Geometry: final body of the model. Coordinates: model frame, mm. Face numbers are marked on the shaded views. A direction names the side the tool comes from. Round coordinates to 2 decimals unless told otherwise and drop trailing zeros. Order: outer loops, then holes, each group sorted by start corner. A loop starts at its lowest first (then second) coordinate and runs counter-clockwise, first axis right, second up. Notation, with made-up numbers: (-15.75, -16.75) -> (16.25, -16.75) arc R5 ccw to (16.25, -8.75) -> close; hole circle Ø4 at (-17, 27.5). An arc over 180 degrees is marked (long way). Put each result on its own line as item: value.
```python
from build123d import *

# Parameters (mm, degrees)
EXTRUDE_1_DEPTH     = 4
EXTRUDE_START       = 2
EXTRUDE_2_DEPTH     = 2
EXTRUDE_3_DEPTH     = 2
SKETCH_4_R          = 1.6
CUT_EXTRUDE_1_DEPTH = 10
CUT_EXTRUDE_2_DEPTH = 3
SKETCH_7_R          = 1.6
CUT_EXTRUDE_3_DEPTH = 10
CUT_EXTRUDE_4_DEPTH = 3


with BuildPart() as part:
    # 草图1 → 凸台-拉伸1 (new body)
    with BuildSketch(Plane.XY):
        with BuildLine():
            Line((-35.40625, 64.537081934), (4.59375, 64.537081934))
            ThreePointArc((4.59375, 64.537081934), (10.957711031, 61.901042965), (13.59375, 55.537081934))
            Line((13.59375, 55.537081934), (13.59375, 15.537081934))
            ThreePointArc((13.59375, 15.537081934), (10.957711031, 9.173120903), (4.59375, 6.537081934))
            Line((4.59375, 6.537081934), (-35.40625, 6.537081934))
            ThreePointArc((-35.40625, 6.537081934), (-41.770211031, 9.173120903), (-44.40625, 15.537081934))
            Line((-44.40625, 15.537081934), (-44.40625, 55.537081934))
            ThreePointArc((-44.40625, 55.537081934), (-41.770211031, 61.901042965), (-35.40625, 64.537081934))
        make_face()
    extrude(amount=-EXTRUDE_1_DEPTH)

    # 草图2 → 凸台-拉伸2 (add)
    with BuildSketch(Plane.XY.offset(EXTRUDE_START)):
        with BuildLine():
            Line((13.59375, 15.537081934), (13.59375, 55.537081934))
            ThreePointArc((13.59375, 55.537081934), (10.957711031, 61.901042965), (4.59375, 64.537081934))
            Line((4.59375, 64.537081934), (-35.40625, 64.537081934))
            ThreePointArc((-35.40625, 64.537081934), (-41.770211031, 61.901042965), (-44.40625, 55.537081934))
            Line((-44.40625, 55.537081934), (-44.40625, 15.537081934))
            ThreePointArc((-44.40625, 15.537081934), (-41.770211031, 9.173120903), (-35.40625, 6.537081934))
            Line((-35.40625, 6.537081934), (4.59375, 6.537081934))
            ThreePointArc((4.59375, 6.537081934), (10.957711031, 9.173120903), (13.59375, 15.537081934))
        make_face()
        with BuildLine():
            Line((-35.40625, 63.537081934), (-25.40625, 63.537081934))
            Line((-25.40625, 63.537081934), (-25.40625, 45.537081934))
            Line((-25.40625, 45.537081934), (-43.40625, 45.537081934))
            Line((-43.40625, 45.537081934), (-43.40625, 55.537081934))
            ThreePointArc((-43.40625, 55.537081934), (-41.063104249, 61.193936184), (-35.40625, 63.537081934))
        make_face(mode=Mode.SUBTRACT)
        with BuildLine():
            Line((12.59375, 55.537081934), (12.59375, 45.537081934))
            Line((12.59375, 45.537081934), (-5.40625, 45.537081934))
            Line((-5.40625, 45.537081934), (-5.40625, 63.537081934))
            Line((-5.40625, 63.537081934), (4.59375, 63.537081934))
            ThreePointArc((4.59375, 63.537081934), (10.250604249, 61.193936184), (12.59375, 55.537081934))
        make_face(mode=Mode.SUBTRACT)
        with BuildLine():
            Line((-35.40625, 7.537081934), (-25.40625, 7.537081934))
            Line((-25.40625, 7.537081934), (-25.40625, 25.537081934))
            Line((-25.40625, 25.537081934), (-43.40625, 25.537081934))
            Line((-43.40625, 25.537081934), (-43.40625, 15.537081934))
            ThreePointArc((-43.40625, 15.537081934), (-41.063104249, 9.880227685), (-35.40625, 7.537081934))
        make_face(mode=Mode.SUBTRACT)
        with BuildLine():
            Line((-5.40625, 25.537081934), (12.59375, 25.537081934))
            Line((12.59375, 25.537081934), (12.59375, 15.537081934))
            ThreePointArc((12.59375, 15.537081934), (10.250604249, 9.880227685), (4.59375, 7.537081934))
            Line((4.59375, 7.537081934), (-5.40625, 7.537081934))
            Line((-5.40625, 7.537081934), (-5.40625, 25.537081934))
        make_face(mode=Mode.SUBTRACT)
    extrude(amount=-EXTRUDE_2_DEPTH)

    # 草图3 → 凸台-拉伸3 (add)
    with BuildSketch(Plane.XY.offset(2).offset(EXTRUDE_START)):
        with BuildLine():
            Line((13.59375, 15.537081934), (13.59375, 55.537081934))
            ThreePointArc((13.59375, 55.537081934), (10.957711031, 61.901042965), (4.59375, 64.537081934))
            Line((4.59375, 64.537081934), (-35.40625, 64.537081934))
            ThreePointArc((-35.40625, 64.537081934), (-41.770211031, 61.901042965), (-44.40625, 55.537081934))
            Line((-44.40625, 55.537081934), (-44.40625, 15.537081934))
            ThreePointArc((-44.40625, 15.537081934), (-41.770211031, 9.173120903), (-35.40625, 6.537081934))
            Line((-35.40625, 6.537081934), (4.59375, 6.537081934))
            ThreePointArc((4.59375, 6.537081934), (10.957711031, 9.173120903), (13.59375, 15.537081934))
        make_face()
        with BuildLine():
            Line((-43.40625, 55.537081934), (-43.40625, 45.537081934))
            Line((-43.40625, 45.537081934), (-43.40625, 25.537081934))
            Line((-43.40625, 25.537081934), (-43.40625, 15.537081934))
            ThreePointArc((-43.40625, 15.537081934), (-41.063104249, 9.880227685), (-35.40625, 7.537081934))
            Line((-35.40625, 7.537081934), (-25.40625, 7.537081934))
            Line((-25.40625, 7.537081934), (-5.40625, 7.537081934))
            Line((-5.40625, 7.537081934), (4.59375, 7.537081934))
            ThreePointArc((4.59375, 7.537081934), (10.250604249, 9.880227685), (12.59375, 15.537081934))
            Line((12.59375, 15.537081934), (12.59375, 25.537081934))
            Line((12.59375, 25.537081934), (12.59375, 45.537081934))
            Line((12.59375, 45.537081934), (12.59375, 55.537081934))
            ThreePointArc((12.59375, 55.537081934), (10.250604249, 61.193936184), (4.59375, 63.537081934))
            Line((4.59375, 63.537081934), (-5.40625, 63.537081934))
            Line((-5.40625, 63.537081934), (-25.40625, 63.537081934))
            Line((-25.40625, 63.537081934), (-35.40625, 63.537081934))
            ThreePointArc((-35.40625, 63.537081934), (-41.063104249, 61.193936184), (-43.40625, 55.537081934))
        make_face(mode=Mode.SUBTRACT)
    extrude(amount=-EXTRUDE_3_DEPTH)

    # 草图4 → 切除-拉伸1 (cut)
    with BuildSketch(Plane.XY.offset(2)):
        with Locations((-15.40625, 41.537081934)):
            Circle(SKETCH_4_R)
        with Locations((-15.40625, 29.537081934)):
            Circle(SKETCH_4_R)
        with Locations((4.59375, 35.537081934)):
            Circle(SKETCH_4_R)
        with Locations((-35.40625, 35.537081934)):
            Circle(SKETCH_4_R)
    extrude(amount=-CUT_EXTRUDE_1_DEPTH, mode=Mode.SUBTRACT)

    # 草图5 → 切除-拉伸2 (cut)
    with BuildSketch(Plane.XY.offset(2)):
        Polygon((-13.431907117, 44.024108978), (-16.572907158, 44.490426548), (-18.547250041, 42.003399505), (-17.380592883, 39.050054891), (-14.239592842, 38.58373732), (-12.265249959, 41.070764364), align=None)
        Polygon((1.418323519, 35.537081934), (3.00603676, 32.787081934), (6.18146324, 32.787081934), (7.769176481, 35.537081934), (6.18146324, 38.287081934), (3.00603676, 38.287081934), align=None)
        Polygon((-13.431907117, 27.050054891), (-12.265249959, 30.003399505), (-14.239592842, 32.490426548), (-17.380592883, 32.024108978), (-18.547250041, 29.070764364), (-16.572907158, 26.58373732), align=None)
        Polygon((-32.230823519, 35.537081934), (-33.81853676, 38.287081934), (-36.99396324, 38.287081934), (-38.581676481, 35.537081934), (-36.99396324, 32.787081934), (-33.81853676, 32.787081934), align=None)
    extrude(amount=-CUT_EXTRUDE_2_DEPTH, mode=Mode.SUBTRACT)

    # 草图7 → 切除-拉伸3 (cut)
    with BuildSketch(Plane.XY.offset(2)):
        with Locations((-15.40625, 15.537081934)):
            Circle(SKETCH_7_R)
        with Locations((-15.40625, 55.537081934)):
            Circle(SKETCH_7_R)
    extrude(amount=-CUT_EXTRUDE_3_DEPTH, mode=Mode.SUBTRACT)

    # 草图8 → 切除-拉伸4 (cut)
    with BuildSketch(Plane.XY.offset(2)):
        Polygon((-15.40625, 18.741375928), (-18.18125, 17.139228931), (-18.18125, 13.934934937), (-15.40625, 12.33278794), (-12.63125, 13.934934937), (-12.63125, 17.139228931), align=None)
        Polygon((-15.40625, 58.741375928), (-18.18125, 57.139228931), (-18.18125, 53.934934937), (-15.40625, 52.33278794), (-12.63125, 53.934934937), (-12.63125, 57.139228931), align=None)
    extrude(amount=-CUT_EXTRUDE_4_DEPTH, mode=Mode.SUBTRACT)


solid = part.part
```
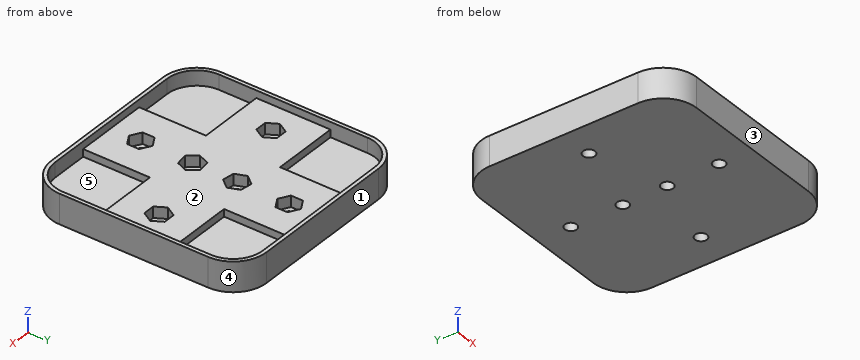
1. Cut plane D-D on x = 9. Return loops of the section in (y, z).
Ans:
outline: (7.69, -4) -> (63.38, -4) -> (63.38, 4) -> (62.21, 4) -> (62.21, 0) -> (45.54, 0) -> (45.54, 2) -> (25.54, 2) -> (25.54, 0) -> (8.86, 0) -> (8.86, 4) -> (7.69, 4) -> close
2. Cut plane A-A on z = 3. Return loops of the section in (x, y).
Ans:
outline: (-44.41, 15.54) arc R9 ccw to (-35.41, 6.54) -> (4.59, 6.54) arc R9 ccw to (13.59, 15.54) -> (13.59, 55.54) arc R9 ccw to (4.59, 64.54) -> (-35.41, 64.54) arc R9 ccw to (-44.41, 55.54) -> close; hole (-43.41, 15.54) arc R8 ccw to (-35.41, 7.54) -> (4.59, 7.54) arc R8 ccw to (12.59, 15.54) -> (12.59, 55.54) arc R8 ccw to (4.59, 63.54) -> (-35.41, 63.54) arc R8 ccw to (-43.41, 55.54) -> close
3. Draft query along Y for the marked faces 1, 2 and 3. Return one class per face: +Y half, -Y half, draft (parallel to the pull), parting line (faces both ways), or undercut.
Ans:
face 1: +Y half
face 2: undercut
face 3: -Y half
4. Set-up query: the marked faces 4 and 5. Return all of +Z, -Z, +X, -X, +Y, -Y with unobstructed straight access to the full face (end or side cutting, diameter ignored); none if empty.
Ans:
face 4: +Z, -Z, +X, +Y
face 5: +Z
5. Cut plane C-C on z = -1.75. Return loops of the section in (x, y), and give its area (3 significant figures).
Ans:
outline: (-44.41, 15.54) arc R9 ccw to (-35.41, 6.54) -> (4.59, 6.54) arc R9 ccw to (13.59, 15.54) -> (13.59, 55.54) arc R9 ccw to (4.59, 64.54) -> (-35.41, 64.54) arc R9 ccw to (-44.41, 55.54) -> close; hole circle Ø3.2 at (-35.41, 35.54); hole circle Ø3.2 at (-15.41, 15.54); hole circle Ø3.2 at (-15.41, 29.54); hole circle Ø3.2 at (-15.41, 41.54); hole circle Ø3.2 at (-15.41, 55.54); hole circle Ø3.2 at (4.59, 35.54)
area: 3,250 mm²
6. Cut plane B-B on y = 23. Return loops of the section in (x, z), and give its area (3 significant figures).
Ans:
outline: (-44.41, -4) -> (13.59, -4) -> (13.59, 4) -> (12.59, 4) -> (12.59, 0) -> (-5.41, 0) -> (-5.41, 2) -> (-25.41, 2) -> (-25.41, 0) -> (-43.41, 0) -> (-43.41, 4) -> (-44.41, 4) -> close
area: 280 mm²
7. Material intervals for probe 1 along X at (y, z) = (51, 1.75); probe 2 along Y at (x, z) = (4, 1); probe 3 along X at (y, z) = (40, 2.5), sorted ascending.
Ans:
probe 1: -44.41 to -43.41, -25.41 to -5.41, 12.59 to 13.59
probe 2: 6.54 to 7.54, 25.54 to 32.79, 38.29 to 45.54, 63.54 to 64.54
probe 3: -44.41 to -43.41, 12.59 to 13.59
8. Contact query for flat-ended pins moving along their axis: P1, Ø10, axis at x = -29, y = 37, coming from the +Z side; P2, Ø9, axis at x = -32.5, y = 19.5, coming from the +Z side; P3, Ø3, axis at x = -34.5, y = 35.5, coming from the +Z side. Output: stop coordinate, or through.
Ans:
P1: z = 2
P2: z = 0
P3: z = -1
